The listing builds one solid part. Answer for the finished solid, in the listing's coordinates (mm). A direction names the side the tool comes from. Give positions to 0.01 mm unless a question says otherwise; leave off trailing zeros. Order: outer loops, then holes, each group sorted by start corner. A loop starts at its lowest first (then second) coordinate and runs counter-clockwise, first axis right, second up. Notation, with made-up numbers: (51, 23) - (75, 23) arc R12 cw to (75, 27) - close; hole circle Ø9 at (33, 81). An arc over 180 degrees is marked (long way). Answer in a Markdown table with one row per item.
Autodesk Inventor part; units mm, degrees
ref_plane "YZ Plane" through (0, 0, 0) normal (1, 0, 0) x (0, 1, 0)
ref_plane "XZ Plane" through (0, 0, 0) normal (0, 1, 0) x (-1, 0, 0)
ref_plane "XY Plane" through (0, 0, 0) normal (0, 0, 1) x (1, 0, 0)
sketch "Sketch2" plane through (0, 0, 0) normal (0, 0, 1) x (1, 0, 0)
  line L0 (0, 0) -> (25.4, 0)
  line L1 (25.4, 0) -> (25.4, 25.4)
  line L2 (25.4, 25.4) -> (0, 25.4)
  line L3 (0, 25.4) -> (0, 0)
  line L4 (23.114, 23.114) -> (23.114, 2.286)
  line L5 (23.114, 2.286) -> (2.286, 2.286)
  line L6 (2.286, 2.286) -> (2.286, 23.114)
  line L7 (2.286, 23.114) -> (23.114, 23.114)
  dimension "d0" = 25.4
  dimension "d1" = 25.4
  dimension "d2" = 2.286
extrude "Extrusion1" add sketch "Sketch2" along normal blind 635
sketch "Sketch3" plane through (25.4, 0, 0) normal (1, 0, 0) x (0, 0, -1)
  circle A0 centre (-12.7, 12.7) radius 2.5527
  line L0 (0, 0) -> (-635, 0)
  line L1 (0, 0) -> (0, 25.4)
  dimension "d5" = 5.1054
  dimension "d6" = 12.7
  dimension "d7" = 12.7
extrude "Extrusion2" cut sketch "Sketch3" against normal blind 609.6
pattern_linear "Rectangular Pattern1" count 25 spacing 25.4 along (0, 0, 1) of "Extrusion2"
sketch "Sketch4" plane through (0, 25.4, 0) normal (0, 1, 0) x (1, 0, 0)
  point P0 (0, 0)
sketch "Sketch5" plane through (0, 25.4, 0) normal (0, 1, 0) x (1, 0, 0)
  circle A0 centre (12.7, -12.7) radius 4.7625
  line L0 (25.4, 0) -> (0, 0)
  line L1 (0, 0) -> (0, -635)
  circle A1 centre (12.7, -116.078) radius 4.7625
  circle A2 centre (12.7, -622.3) radius 4.7625
  circle A3 centre (12.7, -518.922) radius 4.7625
  line L2 (25.4, -635) -> (0, -635)
  line L3 (25.4, 0) -> (25.4, -635)
  point P0 (12.7, 0)
  dimension "d13" = 12.7
  dimension "d14" = 12.7
  dimension "d15" = 9.525
  dimension "d16" = 9.525
  dimension "d17" = 103.378
  dimension "d18" = 12.7
  dimension "d19" = 9.525
  dimension "d20" = 9.525
  dimension "d21" = 103.378
  dimension "d22" = 12.7
  dimension "d23" = 12.7
  dimension "d24" = 12.7
extrude "Extrusion3" cut sketch "Sketch5" against normal blind 635 contours A0 | A1 | A2 | A3
properties part number "Leg_tube"
Item 1: Determine the mould class of faces 1 (the face through (13, 2.286, 313)), 2 (the face through (24, 13, 635)), 3 (the face through (0, 13, 313)), 4 (the face through (23.114, 13, 313)) for opening direction X: pulls with the +X half, pulls with the -X half, needs draft (parallel to the pull), parting line crosses it, or undercut.
Answer block:
| item | result |
|---|---|
| face 1 | undercut |
| face 2 | needs draft |
| face 3 | pulls with the -X half |
| face 4 | undercut |
Item 2: This flat-tipped pin is pushed along its axis until it touches: P1, Ø6.5, axis at y = 12.7, z = 444.5, coming from the +X side. Where does it stop, or does it pass through?
Answer block:
| item | result |
|---|---|
| P1 | x = 25.4 |
Item 3: Find section B-B on x = 12.7. Count the separate pieces of the cut face and the enclosed holes in it, then the cut area to 3 significant figures.
Answer block:
| item | result |
|---|---|
| separate pieces | 10 |
| enclosed holes | 0 |
| area | 2,730 mm² |
Item 4: Which of the six approach directions +Z, -Z, +X, -X, +Y, -Y give full straight-line access (tool end or side, diameter ignored) to faces 5 (the face through (25.4, 13, 313)), 6 (the face through (13, 23.114, 313))?
Answer block:
| item | result |
|---|---|
| face 5 | +Z, -Z, +X, +Y, -Y |
| face 6 | +Z, -Z |
Item 5: Find section A-A on z = 131.5. Write down the section's boundary in (x, y).
Answer block:
| item | result |
|---|---|
| outline | (0, 0) - (25.4, 0) - (25.4, 25.4) - (0, 25.4) - close; hole (2.29, 2.29) - (23.11, 2.29) - (23.11, 23.11) - (2.29, 23.11) - close |
Item 6: Consider line 1 (Z direction, x = 12.7, y = 0.85); line 2 (Y direction, x = 12.5, z = 302); line 3 (Y direction, x = 23.95, z = 419.1). Determine where each line is inside the solid, lowest interval first.
Answer block:
| item | result |
|---|---|
| line 1 | 0 to 7.94, 17.46 to 111.32, 120.84 to 514.16, 523.68 to 617.54, 627.06 to 635 |
| line 2 | 0 to 2.29, 23.11 to 25.4 |
| line 3 | 0 to 10.15, 15.25 to 25.4 |
